Input: part model. Units: mm. Frame: model coordinates. A direction names the side the tool comes from. Give positions to 0.01 mm unless a question says otherwise; leave off trailing zeros. Loops run counter-clockwise (first coordinate to the right, second up) from the corner with the lowest first, then second, coordinate; pieces in that order, holes last. Notation, with made-up numbers: M 56,-22 L 74,-22 A20 ccw 74,-4 Z; hole C -30.5,84.5 d8. An arc over 180 degrees is marked long. Return JSON: item names as keys, results as strings. Group by question number.
```python
from build123d import *

# Parameters (mm, degrees)
F1_DEPTH = 10.033
F3_DEPTH = 76.2
F4_W     = 6.35
F4_H     = 6.35
F5_DEPTH = 76.2
F7_D     = 2.2606
F7_DEPTH = 8.255
F7_TIP   = 0.6791527577
F9_D     = 2.2606
F9_DEPTH = 8.255
F9_TIP   = 0.6791527577


with BuildPart() as f1:
    # F0 (on Right) → F1 (new body, symmetric)
    with BuildSketch(Plane.YZ):
        Polygon((19.05, -6.35), (31.75, 6.35), (-19.05, 6.35), (-31.75, -6.35), align=None)
    extrude(amount=F1_DEPTH, both=True)

    # F2 (on Front) → F3 (cut, symmetric)
    with BuildSketch(Plane.XZ):
        Polygon((-6.858, -3.81), (-5.588, -6.35), (5.588, -6.35), (6.858, -3.81), align=None)
        Polygon((5.588, 6.35), (-5.588, 6.35), (-6.858, 3.81), (6.858, 3.81), align=None)
    extrude(amount=F3_DEPTH, both=True, mode=Mode.SUBTRACT)

    # F4 (on Front) → F5 (cut, symmetric)
    with BuildSketch(Plane.XZ):
        with Locations((6.858, 3.175)):
            Rectangle(F4_W, F4_H)
        with Locations((-6.858, -3.175)):
            Rectangle(F4_W, F4_H)
    extrude(amount=F5_DEPTH, both=True, mode=Mode.SUBTRACT)

    # F7
    with Locations(Plane.YZ.offset(3.683)):
        with Locations((-9.525, 1.905), (15.875, 1.905)):
            Hole(F7_D / 2, depth=F7_DEPTH)
            with Locations((0, 0, -(F7_DEPTH + F7_TIP / 2))):  # 118° drill point
                Cone(0, F7_D / 2, F7_TIP, mode=Mode.SUBTRACT)

    # F9
    with Locations(Plane(origin=(-3.683, 0, 0), x_dir=(0, -1, 0), z_dir=(-1, 0, 0))):
        with Locations((-9.525, -1.905), (15.875, -1.905)):
            Hole(F9_D / 2, depth=F9_DEPTH)
            with Locations((0, 0, -(F9_DEPTH + F9_TIP / 2))):  # 118° drill point
                Cone(0, F9_D / 2, F9_TIP, mode=Mode.SUBTRACT)


solid = f1.part
```
Item 1: Section A-A, the plane x = 2.5. Return loops of the section in (y, z) (3 decimals).
Item 2: First-contact query: pin 1 Ø3 at (x, y) = (5.5, 4.5) entering from +Z; pin 2 Ø2 at (y, z) = (9.525, -1.905) entering from -X; pin 3 Ø1 at (x, y) = (-4, 14.5) entering from -Z. Flat tips, straight axial feed; report the tip coordinate or a pass-through.
Item 3: Section D-D, the plane z = 5.5. Return loops of the section in (x, y), then the cut area to 3 significant figures.
Item 4: Pull-direction query (Z, two-part tool) for faces 1 (the face through (7, 0, 0)), 2 (the face through (-5.133, 15.679, 1.914)), 3 (the face through (-7, 0, 0)), 4 (the face through (-6.214, 4.707, 5.098)); classes: pulls with the +Z half, pulls with the -Z half, needs draft (parallel to the pull), parting line crosses it, or undercut.
Item 5: Material intervals for line 1 (Y direction, x = -2.25, z = 1.5); line 2 (Z direction, x = 0.25, y = 3); line 3 (Y direction, x = -5, z = 1.75), sorted ascending. Write a range as from..to.
Item 6: Section B-B, the plane y = 0.5. Return loops of the section in (x, z).
Item 7: Section C-C, the plane x = -8.5. Return loops of the section in (y, z), then the cut area to 3 significant figures.
Item 8: Reachability of faces 5 (the face through (6.214, -4.707, -5.098)), 6 (the face through (-0.502, -8.692, 2.669)), 7 (the face through (1, -17, -2)) from +Z, -Z, +X, -X, +Y, -Y: full face, straight path, thin tool, end or side. Return the list, or none.
Answer below:
{
 "1": {"outline": "M -29.21,-3.81 L 21.59,-3.81 L 29.21,3.81 L -21.59,3.81 Z; hole C -15.875,-1.905 d2.261; hole C -9.525,1.905 d2.261; hole C 9.525,-1.905 d2.261; hole C 15.875,1.905 d2.261"},
 "2": {"pin 1": "z = 0", "pin 2": "x = 4.65", "pin 3": "z = -3.81"},
 "3": {"outline": "M -10.03,-19.9 L -6.01,-19.9 L -6.01,30.9 L -10.03,30.9 Z", "area": "204 mm^2"},
 "4": {"face 1": "pulls with the +Z half", "face 2": "undercut", "face 3": "pulls with the -Z half", "face 4": "undercut"},
 "5": {"line 1": "-23.9..-10.58, -8.47..14.82, 16.93..26.9", "line 2": "-3.81..3.81", "line 3": "-23.65..-9.91, -9.14..15.49, 16.26..27.15"},
 "6": {"outline": "M -10.03,0 L -3.68,0 L -3.68,-3.81 L 6.86,-3.81 L 5.59,-6.35 L 10.03,-6.35 L 10.03,0 L 3.68,0 L 3.68,3.81 L -6.86,3.81 L -5.59,6.35 L -10.03,6.35 Z"},
 "7": {"outline": "M -25.4,0 L 25.4,0 L 31.75,6.35 L -19.05,6.35 Z", "area": "323 mm^2"},
 "8": {"face 5": "-X, +Y, -Y", "face 6": "+X", "face 7": "-X"}
}
